Check sheet for the drawn part. Datum: minimum x, y, z corner. Units: mm. A direction names the side the tool comes from. Coordinates: 2 decimals unless noted, no trailing zeros. Write each loop counter-clockwise with the first axis right and the second up, starting at its lowest first coordinate (ties: lowest second). Pieces come first, ordered by that corner, then holes. Notation, with made-up numbers: M -18.75,59 L 37.25,59 A15 ccw 37.25,69 Z; hole C -33,17.25 d3. An arc over 180 degrees is marked long. Answer as a JSON object with one key per item and string values. Group by question number.
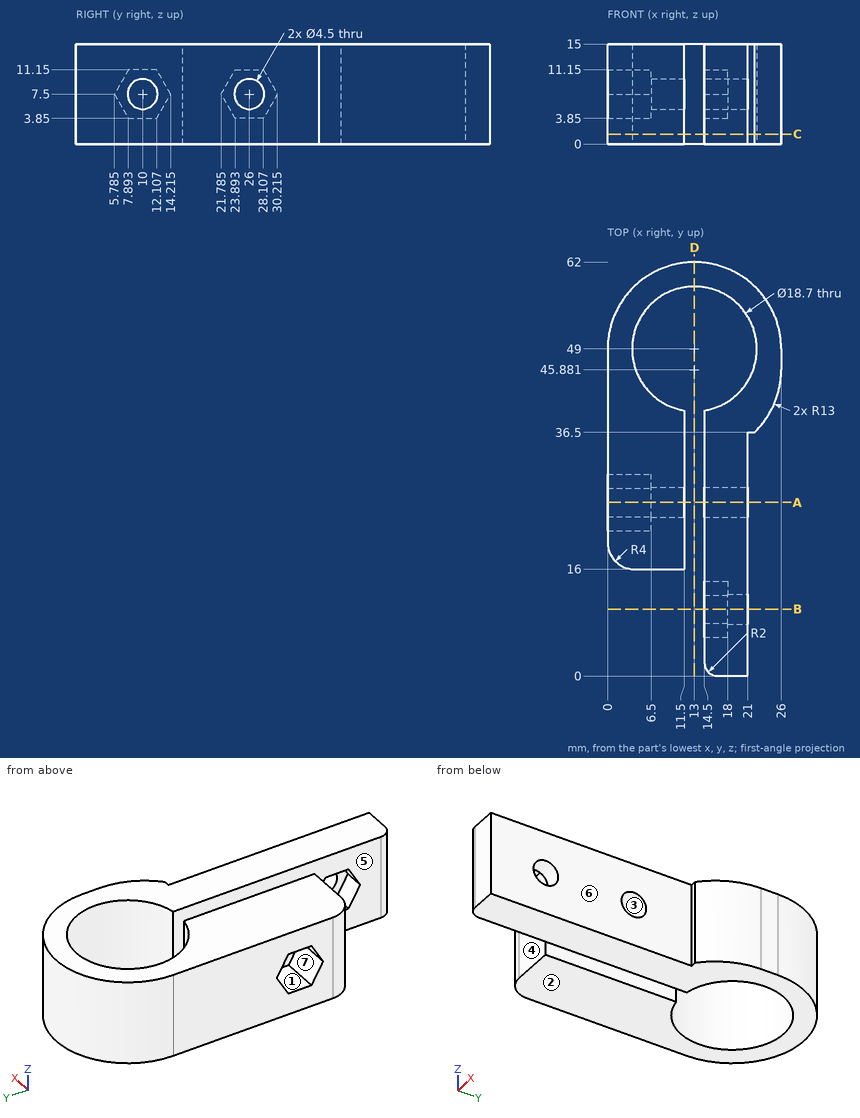
1) Section check B-B (y = 10). Record the cut outline in (x, z).
2) Set-up check for the marked faces 5, 6 and 7: record each of +Z, -Z, +X, -X, +Y, -Y from which the full face is reachable in a straight line by a thin tool's end or side.
3) Section check D-D (x = 13). Record the cut outline in (y, z).
4) Go/stop test with flat-tipped pins: pin 1 Ø2 at (x, z) = (7, 8) entering from -Y; pin 2 Ø8 at (y, z) = (11.5, 6) entering from -X; pin 3 Ø5 at (y, z) = (37, 10.5) entering from +X. Record where each tip stops, or that it passes through.
5) Section check C-C (z = 1.5). Record the cut outline in (x, y).
6) Material ranges on probe 1 along X at (y, z) = (22, 13.5); probe 2 along Y at (x, z) = (19.45, 7.5); probe 3 along X at (y, z) = (49.5, 13), recorded low to high. Write a range as [from, to].
7) Section check A-A (y = 26). Record the cut outline in (x, z).
8) Draft check along Y on the marked faces 1, 2, 3 and 4. Enter one of: +Y half, -Y half, draft (parallel to the pull), parting line (faces both ways), or undercut.
Entries:
{
 "1": {"outline": "M 14.5,0 L 21,0 L 21,5.25 L 18,5.25 L 18,3.85 L 14.5,3.85 Z; M 14.5,11.15 L 18,11.15 L 18,9.75 L 21,9.75 L 21,15 L 14.5,15 Z"},
 "2": {"face 5": "+Z, -Z, -Y", "face 6": "+Z, -Z, +X, -Y", "face 7": "-X"},
 "3": {"outline": "M 58.35,0 L 62,0 L 62,15 L 58.35,15 Z"},
 "4": {"pin 1": "y = 16", "pin 2": "x = 14.5", "pin 3": "x = 24.33"},
 "5": {"outline": "M 0,20 A4 ccw 4,16 L 11.5,16 L 11.5,39.77 A9.35 cw long 14.5,39.77 L 14.5,2 A2 ccw 16.5,0 L 21,0 L 21,36.5 L 22,36.5 A13 ccw 26,45.88 L 26,49 A13 ccw 0,49 Z"},
 "6": {"probe 1": "[0, 11.5], [14.5, 21]", "probe 2": "[0, 7.75], [12.25, 23.75], [28.25, 42.23], [55.77, 60.29]", "probe 3": "[0.01, 3.66], [22.34, 25.99]"},
 "7": {"outline": "M 0,0 L 11.5,0 L 11.5,5.25 L 6.5,5.25 L 6.5,3.85 L 0,3.85 Z; M 0,11.15 L 6.5,11.15 L 6.5,9.75 L 11.5,9.75 L 11.5,15 L 0,15 Z; M 14.5,0 L 21,0 L 21,5.25 L 14.5,5.25 Z; M 14.5,9.75 L 21,9.75 L 21,15 L 14.5,15 Z"},
 "8": {"face 1": "undercut", "face 2": "draft", "face 3": "undercut", "face 4": "-Y half"}
}
